CAD build for the part. Positions are in the model's coordinates, mm. A direction names the side the tool comes from. Give positions to 0.01 mm unless a question says otherwise; leave off trailing zeros. Loops run counter-clockwise (first coordinate to the right, second up) from the corner with the lowest first, then second, coordinate; pieces in that order, holes last. Notation, with made-up numbers: M 15.25,16 L 64.25,16 A20 cw 64.25,39 Z; hole C -29.75,9.25 d6. An arc over 180 degrees is marked long. One line per question, with ' | ' between items.
```python
from build123d import *

# Parameters (mm, degrees)
F0_W     = 25
F0_H     = 15
F1_DEPTH = 7
F3_W     = 2
F3_H     = 10
F4_DEPTH = 5
F5_W     = 2
F5_H     = 10
F6_DEPTH = 5
F9_D     = 2


with BuildPart() as f1:
    # F0 (on Top) → F1 (new body)
    with BuildSketch(Plane.XY):
        with Locations((12.5, 7.5)):
            Rectangle(F0_W, F0_H)
    extrude(amount=F1_DEPTH)

    # F3 (on face) → F4 (join)
    with BuildSketch(Plane.XY.offset(7)):
        with Locations((1, 5)):
            Rectangle(F3_W, F3_H)
    extrude(amount=F4_DEPTH)

    # F5 (on face) → F6 (join)
    with BuildSketch(Plane.XY.offset(7)):
        with Locations((23.98319, 5)):
            Rectangle(F5_W, F5_H)
    extrude(amount=F6_DEPTH)

    # F9 (through all)
    with Locations(Plane.XY.offset(7)):
        with Locations((7.460146, 8.077994), (17.4512, 8.020776)):
            Hole(F9_D / 2)


solid = f1.part
```
Item 1: Mould opens along X. For faces 4 (the flat face through (22.983, 5, 9)), 5 (the flat face through (25, 7, 3)), 6 (the flat face through (24, 10, 9)) say: pulls with the +X half, pulls with the -X half, needs draft (parallel to the pull), parting line crosses it, or undercut.
Conclusion:
face 4: undercut | face 5: pulls with the +X half | face 6: needs draft
Item 2: Saw through at C-C on z = 2.75. Give the cut face in (x, y), and give its area (3 significant figures).
Conclusion:
outline: M 0,0 L 25,0 L 25,15 L 0,15 Z; hole C 7.46,8.08 d2; hole C 17.45,8.02 d2 | area: 369 mm²
Item 3: Saw through at B-B on x = 7. Give the cut face in (y, z).
Conclusion:
outline: M 0,0 L 7.19,0 L 7.19,7 L 0,7 Z; M 8.97,0 L 15,0 L 15,7 L 8.97,7 Z
Item 4: 3-axis set-ups, long thin cutter, end or side, ignore diameter. For faces 1 (the cylindrical face through (8.46, 8.12, 3.45)), 2 (the flat face through (2, 5, 9)), 3 (the flat face through (1, 10, 9)): which of +Z, -Z, +X, -X, +Y, -Y reach the whole face in a straight line?
Conclusion:
face 1: +Z, -Z | face 2: +Z, +Y, -Y | face 3: +Z, +X, -X, +Y
Item 5: Drop flat-ended pins along their axis: P1, Ø2.5, axis at y = 7, z = 10, coming from the +X side; P2, Ø2, axis at x = 1.5, z = 10.5, coming from the +Y side; P3, Ø8, axis at x = 13.5, y = 4.5, coming from the +Z side; P4, Ø2, axis at y = 12.5, z = 3, coming from the -X side. Give the stop position or say it passes through.
Conclusion:
P1: x = 24.98 | P2: y = 10 | P3: z = 7 | P4: x = 0
Item 6: Drill centre lines: line 1 along X through (y, z) = (8, 3); line 2 along X through (y, z) = (6.5, 9.25); line 3 along Z through (x, y) = (1.75, 13). Where is each one in solid material? Low to high. Write a range as [from, to].
Conclusion:
line 1: [0, 6.46], [8.46, 16.45], [18.45, 25] | line 2: [0, 2], [22.98, 24.98] | line 3: [0, 7]
Item 7: Saw through at D-D on x = 19.25. Give the cut face in (y, z).
Conclusion:
outline: M 0,0 L 15,0 L 15,7 L 0,7 Z
